Geometry: final body of the model. Coordinates: model frame, mm. Face numbers are marked on the shaded views. A direction names the side the tool comes from. Coordinates: 2 decimals unless noted, no trailing zeros. Loops run counter-clockwise (first coordinate to the right, second up) from the corner with the lowest first, then second, coordinate; pieces in that order, holes last. Notation, with made-up numbers: (40, 38.25) - (76, 38.25) arc R30 ccw to (76, 77.25) - close; hole circle Ø8 at (49, -20). An arc over 180 degrees is marked (long way). Write each question's results on one line, items separated by ' | '. Start each with the question number.
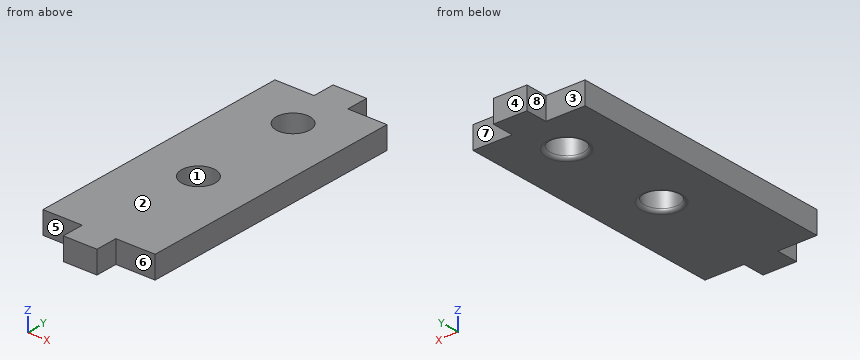
Autodesk Inventor part; units mm, degrees
ref_plane "YZ Plane" through (0, 0, 0) normal (1, 0, 0) x (0, 1, 0)
ref_plane "XZ Plane" through (0, 0, 0) normal (0, 1, 0) x (-1, 0, 0)
ref_plane "XY Plane" through (0, 0, 0) normal (0, 0, 1) x (1, 0, 0)
sketch "Sketch1" plane through (0, 0, 0) normal (0, 0, 1) x (1, 0, 0)
  line L0 (0, 0) -> (100, 0)
  line L1 (100, 0) -> (100, 285)
  line L2 (100, 285) -> (0, 285)
  line L3 (0, 285) -> (0, 0)
  dimension "d0" = 100
  dimension "d1" = 285
extrude "Extrusion1" add sketch "Sketch1" along normal blind 20
sketch "Sketch2" plane through (0, 0, 0) normal (0, 0, -1) x (-1, 0, 0)
  circle A0 centre (-50, 125) radius 15
  circle A1 centre (-50, 225) radius 15
  line L0 (0, 285) -> (0, 0)
  line L1 (0, 0) -> (-100, 0)
  dimension "d5" = 30
  dimension "d6" = 50
  dimension "d7" = 50
  dimension "d9" = 100
  dimension "d13" = 125
extrude "Extrusion2" cut sketch "Sketch2" against normal up to next
sketch "Sketch3" plane through (0, 0, 20) normal (0, 0, 1) x (1, 0, 0)
  line L0 (0, 0) -> (100, 0)
  line L1 (100, 285) -> (0, 285)
  line L2 (35, 285) -> (35, 265)
  line L3 (0, 285) -> (0, 0)
  line L4 (100, 0) -> (100, 285)
  line L5 (35, 265) -> (0, 265)
  line L6 (65, 285) -> (65, 265)
  line L7 (65, 265) -> (100, 265)
  line L8 (35, 0) -> (35, 20)
  line L9 (35, 20) -> (0, 20)
  line L10 (65, 0) -> (65, 20)
  line L11 (100, 20) -> (65, 20)
  dimension "d14" = 30
  dimension "d26" = 35
  dimension "d27" = 20
  dimension "d28" = 20
extrude "Extrusion3" cut sketch "Sketch3" against normal up to next contours L3 L9 L8 L0 | L10 L11 L4 L0 | L3 L1 L2 L5 | L7 L6 L1 L4
sketch "Sketch5" plane through (100, 20, 0) normal (1, 0, 0) x (0, 0, -1)
  line L0 (-20, 0) -> (-20, 245)
  line L1 (-20, 122.5) -> (-90.7107, 193.2107) construction
  line L2 (-20, 122.5) -> (80, 122.5) construction
  line L3 (-20, 265) -> (0, 265)
  point P0 (0, -20)
  dimension "d21" = 100
  dimension "d22" = 135
  dimension "d23" = 142.5
fillet "Fillet1" radius 3 2 edges at (65, 125, 0) (65, 225, 0)
properties part number "MidjuHaldarar" material "Wood (Birch)"
1) Section query A-A on y = 225. Output: boundary loops of the cut face in (x, z).
2) Access query for the marked faces 4, 5, 6, 7 and 8. Directions: +Z, -Z, +X, -X, +Y, -Y. A direction counts if a zero-diameter tool reaches every point of the face in a straight line with its end or side. Return the directions, or none.
3) Pin query (flat end, axial travel): pin 1 Ø2 at (x, z) = (33, 13.5) entering from -Y; pin 2 Ø12 at (y, z) = (46.5, 6.5) entering from -X; pin 3 Ø5 at (x, z) = (17, 17) entering from +Y; pin 4 Ø10 at (y, z) = (11, 11.5) entering from -X. Return the tip coordinate at first contact, or that it passes through.
4) Section query D-D on x = 70.5. Output: boundary loops of the cut face in (y, z).
5) Section query B-B on x = 50. Output: boundary loops of the cut face in (y, z), and give its area (3 significant figures).
6) Pull-direction query (Y, two-part tool) for the marked faces 1, 2 and 3; classes: released by +Y, released by -Y, zero draft, split by the parting line, or undercut.
7) Material intervals for line 1 (Y direction, x = 50, z = 14.75); line 2 (Y direction, x = 39, z = 18); line 3 (Y direction, x = 20.5, z = 1), sorted ascending. Write a range as [from, to].
8) Section query C-C on z = 10.5. Output: boundary loops of the cut face in (x, y).
Returned:
1) outline: (0, 0) - (32, 0) arc R3 ccw to (35, 3) - (35, 20) - (0, 20) - close; (65, 3) arc R3 ccw to (68, 0) - (100, 0) - (100, 20) - (65, 20) - close
2) face 4: +Z, -Z, +X, -X, +Y | face 5: +Z, -Z, -X, -Y | face 6: +Z, -Z, +X, -Y | face 7: +Z, -Z, +X, +Y | face 8: +Z, -Z, -X, +Y
3) pin 1: stops at y = 20 | pin 2: stops at x = 0 | pin 3: stops at y = 265 | pin 4: stops at x = 35
4) outline: (20, 0) - (265, 0) - (265, 20) - (20, 20) - close
5) outline: (0, 0) - (107, 0) arc R3 ccw to (110, 3) - (110, 20) - (0, 20) - close; (140, 3) arc R3 ccw to (143, 0) - (207, 0) arc R3 ccw to (210, 3) - (210, 20) - (140, 20) - close; (240, 3) arc R3 ccw to (243, 0) - (285, 0) - (285, 20) - (240, 20) - close | area: 4,490 mm²
6) face 1: undercut | face 2: zero draft | face 3: released by +Y
7) line 1: y = [0, 110], [140, 210], [240, 285] | line 2: y = [0, 114.8], [135.2, 214.8], [235.2, 285] | line 3: y = [20, 265]
8) outline: (0, 20) - (35, 20) - (35, 0) - (65, 0) - (65, 20) - (100, 20) - (100, 265) - (65, 265) - (65, 285) - (35, 285) - (35, 265) - (0, 265) - close; hole circle Ø30 at (50, 125); hole circle Ø30 at (50, 225)
